```python
from build123d import *

# Parameters (mm, degrees)
F1_ANGLE = 143.2394
F2_SIZE2 = 1.999
F2_SIZE  = 1.999


# Not quite as in the source:
# - a fillet or chamfer is up to 0.001 mm smaller than in the source, because OpenCascade refuses the exact size
# - a feature names something its author has since deleted; it is built from what else it names


with BuildPart() as f1:
    # F0 (on Front) → F1 (revolve)
    with BuildSketch(Plane.XZ):
        Polygon((23.4142135624, 0), (38.9705627485, 15.5563491861), (37.5563491861, 16.9705627485), (22, 1.4142135624), align=None)
    revolve(axis=Axis((0, 0, 11), (0, 0, 1)), revolution_arc=F1_ANGLE)

    # F2 (size 2 and 2 in the source; OpenCascade refuses exactly that, so slightly less here)
    f2_edges = [f1.edges().sort_by_distance(p)[0] for p in [
        (11.842372, 35.640393, 16.970563),
    ]]
    chamfer(f2_edges, length=F2_SIZE, length2=F2_SIZE2)


solid = f1.part
```
The listing builds one solid part. Answer for the finished solid, in the listing's coordinates (mm). Give positions to 0.01 mm unless a question says otherwise; leave off trailing zeros. Order: outer loops, then holes, each group sorted by start corner. A loop starts at its lowest first (then second) coordinate and runs counter-clockwise, first axis right, second up. Notation, with made-up numbers: (-15, -18.5) -> (5, -18.5) arc R30 ccw to (5, 9.5) -> close; hole circle Ø3 at (74, 64). An arc over 180 degrees is marked (long way). Answer as a JSON object with one key per item and string values. Group by question number.
Item 1: The part is cut by section A-A on z = 5.75. Write down the section's boundary in (x, y).
Item 2: Consider L1, parallel to X at y = 22, z = 9.75; L2, parallel to X at y = 21, z = 9; L3, parallel to Y at x = -15, z = 13. Determine where each line is inside the solid, lowest interval first. Write a range as from..to.
Item 3: The part is cut by section B-B on z = 12. Write down the section's boundary in (x, y).
Item 4: Flat-ended cylindrical pins translate along their axes: pin 1 (8 mm diameter, centred on x = 1, z = 10, fed in from +Y); pin 2 (1 mm diameter, centred on x = -13, z = 9.5, fed in from +Y); pin 3 (6 mm diameter, centred on x = 29, z = 5, fed in from -Y); pin 4 (4 mm diameter, centred on x = 21, z = 3.5, fed in from +Y). Find the tip coordinate at first contact, or state that the pin passes through.
Item 5: Determine the mould class of faces 1 (the flat face through (30, 0, 8)), 2 (the conical face through (9.241, 26.266, 4.43)), 3 (the flat face through (-23.888, 17.845, 8.391)), 4 (the conical face through (7.383, 20.985, 1.169)) for opening direction X: pulls with the +X half, pulls with the -X half, needs draft (parallel to the pull), parting line crosses it, or undercut.
Result set:
{
 "1": {"outline": "(-23.36, 17.45) -> (-21.1, 15.76) arc R26.34 cw to (26.34, 0) -> (29.16, 0) arc R29.16 ccw to start"},
 "2": {"L1": "-24.82..-20.89, 20.89..24.82", "L2": "-24.69..-20.84, 20.84..24.69", "L3": "30.05..33.18"},
 "3": {"outline": "(-28.37, 21.19) -> (-26.11, 19.5) arc R32.59 cw to (32.59, 0) -> (35.41, 0) arc R35.41 ccw to start"},
 "4": {"pin 1": "y = 37.4", "pin 2": "y = 30.82", "pin 3": "y = 0", "pin 4": "y = 20.52"},
 "5": {"face 1": "needs draft", "face 2": "parting line crosses it", "face 3": "pulls with the -X half", "face 4": "undercut"}
}
